Geometry: final body of the model. Coordinates: model frame, mm. Face numbers are marked on the shaded views. A direction names the side the tool comes from. Coordinates: 2 decimals unless noted, no trailing zeros. Write each loop counter-clockwise with the first axis right and the second up, starting at its lowest first coordinate (ties: lowest second). Pieces come first, ordered by that corner, then holes. Notation, with made-up numbers: (2, 13) - (40, 13) arc R6 ccw to (40, 22) - close; hole circle Ø8 at (-28, 74). An arc over 180 degrees is marked (long way). Answer as a JSON object with one key per item and string values. Group by question number.
Item 1: Line query: line 1 along Z through (x, y) = (12.5, -41); line 2 along Z through (x, y) = (-168, -740.5); line 3 along X through (y, z) = (-164, 128). Output: solid intervals per line, ascending. Write a range as from..to.
Item 2: First-contact query: pin 1 Ø1 at (x, y) = (-133.5, -658) entering from -Z. Flat tip, straight axial feed; report the tip coordinate or a pass-through.
Item 3: Section A-A on y = -22.5. Return loops of the section in (x, z), and give its area (3 significant figures).
Item 4: Section B-B on x = -75.5. Return loops of the section in (y, z).
Item 5: Mould query, pull axis X, two halves, no side actions, for the marked faces 3, 4 and 5. Classes: pulls with the +X half, pulls with the -X half, needs draft (parallel to the pull), parting line crosses it, or undercut.
Item 6: Set-up query: the marked faces 1 and 2. Return all of +Z, -Z, +X, -X, +Y, -Y with unobstructed straight access to the full face (end or side cutting, diameter ignored); none if empty.
Item 7: Section C-C on z = -223.5. Return loops of the section in (x, y), and give its area (3 significant figures).
Item 8: Section D-D on y = -623. Return loops of the section in (x, z).
```python
from build123d import *

# Parameters (mm, degrees)
F1_DEPTH = 200
F2_DEPTH = 1800
F3_DEPTH = 200


with BuildPart() as f1:
    # F0 (on Front) → F1 (new body)
    with BuildSketch(Plane.XZ):
        Polygon((-150, 183.772751), (-200, 183.772751), (-175, -266.227249), (175, -266.227249), (200, 183.772751), (150, 183.772751), (84.275194, 173.772751), (-94.773179, 163.772751), align=None)
        Polygon((-156.080271, -246.227249), (-178.858048, 163.772751), (-153.509895, 163.772751), (-97.739527, 143.575909), (86.341696, 153.856998), (151.512791, 163.772751), (178.858048, 163.772751), (156.080271, -246.227249), align=None, mode=Mode.SUBTRACT)
    extrude(amount=F1_DEPTH)

    # F0 (on Front) → F2 (join)
    with BuildSketch(Plane.XZ):
        Polygon((-201.214484, 205.517881), (-200, 183.772751), (-150, 183.772751), (150, 183.772751), (200, 183.772751), (199.590698, 205.517881), align=None)
    extrude(amount=F2_DEPTH)

    # F0 (on Front) → F3 (join)
    with BuildSketch(Plane.XZ):
        Polygon((-201.214484, 205.517881), (-200, 183.772751), (-150, 183.772751), (150, 183.772751), (200, 183.772751), (199.590698, 205.517881), align=None)
    extrude(amount=-F3_DEPTH)


solid = f1.part
```
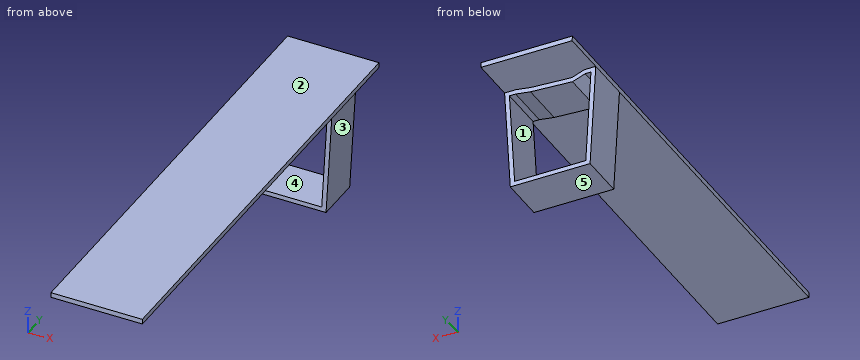
Checks:
{
 "1": {"line 1": "-266.23..-246.23, 149.73..169.76, 183.77..205.52", "line 2": "183.77..205.52", "line 3": "-196.9..-176.87, 176.87..196.9"},
 "2": {"pin 1": "z = 183.77"},
 "3": {"outline": "(-201.21, 205.52) - (-200, 183.77) - (-175, -266.23) - (175, -266.23) - (200, 183.77) - (199.59, 205.52) - close; hole (-178.86, 163.77) - (-156.08, -246.23) - (156.08, -246.23) - (178.86, 163.77) - (151.51, 163.77) - (86.34, 153.86) - (-97.74, 143.58) - (-153.51, 163.77) - close; hole (-150, 183.77) - (-94.77, 163.77) - (84.28, 173.77) - (150, 183.77) - close", "area": "40,200 mm^2"},
 "4": {"outline": "(-1800, 183.77) - (200, 183.77) - (200, 205.52) - (-1800, 205.52) - close; (-200, -266.23) - (0, -266.23) - (0, -246.23) - (-200, -246.23) - close; (-200, 144.82) - (0, 144.82) - (0, 164.85) - (-200, 164.85) - close"},
 "5": {"face 3": "pulls with the +X half", "face 4": "undercut", "face 5": "needs draft"},
 "6": {"face 1": "+Y, -Y", "face 2": "+Z, +X, -X, +Y, -Y"},
 "7": {"outline": "(-177.37, -200) - (-157.34, -200) - (-157.34, 0) - (-177.37, 0) - close; (157.34, -200) - (177.37, -200) - (177.37, 0) - (157.34, 0) - close", "area": "8,010 mm^2"},
 "8": {"outline": "(-201.21, 205.52) - (-200, 183.77) - (200, 183.77) - (199.59, 205.52) - close"}
}
